Here's how the part is built. I have some questions about the finished solid (model axes, mm). A direction names the side the tool comes from. Give positions to 0.01 mm unless a question says otherwise; leave off trailing zeros. Loops run counter-clockwise (first coordinate to the right, second up) from the corner with the lowest first, then second, coordinate; pieces in that order, holes last.
Q1. I need wall thicknesses on line 1 (Y direction, x = -51, z = 2.5); line 2 (X direction, y = -1329.5, z = 13); line 3 (X direction, y = -1317.5, z = 14). Which ranges of each line are inside material? Lowest first, please.
Q2. If we section it at A-A (y = -108): Please give me the cut outline in (x, z).
Q3. We'd pull the mould along X, two halves only. Please class faces 4 (the face through (-69.85, -814, 0)), 5 (the face through (-1, -814, -19.05)), 6 (the face through (-57.15, -1588, 0)): +X half, -X half, draft (parallel to the pull), parting line (faces both ways), or undercut.
Q4. For faces 1 (the face through (31.75, -1588, 0)), 2 (the face through (-57.15, -64, 0)), 3 (the face through (69.85, -814, 0)), which set-ups out of +Z, -Z, +X, -X, +Y, -Y let a thin tool reach every point of the face, with its end or its side?
Q5. Will these pins go through, and if not, where does the flat tip stop? P1, Ø11.5, axis at x = 8, z = -4, coming from the +Y side; P2, Ø3, axis at x = 31.5, z = -8.5, coming from the +Y side; P3, Ø10, axis at x = 0.5, z = -0.5, coming from the -Y side.
Q6. If we section it at B-B (z = -1.5): Please give me the cut outline in (x, y).
Q7. If we section it at C-C (x = -33): Please give me the cut outline in (y, z).
from build123d import *

# Parameters (mm, degrees)
F1_DEPTH = 1651
F2_W     = 88.9
F2_H     = 127
F3_DEPTH = 38.101
F4_W     = 88.9
F4_H     = 127
F5_DEPTH = 38.101


with BuildPart() as f1:
    # F0 (on Front) → F1 (new body)
    with BuildSketch(Plane.XZ):
        with BuildLine():
            ThreePointArc((-69.85, -12.7), (-67.990128, -17.190128), (-63.5, -19.05))
            Line((-63.5, -19.05), (63.5, -19.05))
            ThreePointArc((63.5, -19.05), (67.990128, -17.190128), (69.85, -12.7))
            Line((69.85, -12.7), (69.85, 12.7))
            ThreePointArc((69.85, 12.7), (67.990128, 17.190128), (63.5, 19.05))
            Line((63.5, 19.05), (-63.5, 19.05))
            ThreePointArc((-63.5, 19.05), (-67.990128, 17.190128), (-69.85, 12.7))
            Line((-69.85, 12.7), (-69.85, -12.7))
        make_face()
    extrude(amount=F1_DEPTH)

    # F2 (on face) → F3 (cut, through all)
    with BuildSketch(Plane.XY.offset(19.05)):
        with Locations((-12.7, -63.5)):
            Rectangle(F2_W, F2_H)
    extrude(amount=-F3_DEPTH, mode=Mode.SUBTRACT)

    # F4 (on face) → F5 (cut, through all)
    with BuildSketch(Plane.XY.offset(19.05)):
        with Locations((-12.7, -1587.5)):
            Rectangle(F4_W, F4_H)
    extrude(amount=-F5_DEPTH, mode=Mode.SUBTRACT)


solid = f1.part
Check sheet entries:
1. line 1: y = -1524 to -127
1. line 2: x = -69.84 to 69.84
1. line 3: x = -69.72 to 69.72
2. outline: (-69.85, -12.7) arc R6.35 ccw to (-63.5, -19.05) - (-57.15, -19.05) - (-57.15, 19.05) - (-63.5, 19.05) arc R6.35 ccw to (-69.85, 12.7) - close; (31.75, -19.05) - (63.5, -19.05) arc R6.35 ccw to (69.85, -12.7) - (69.85, 12.7) arc R6.35 ccw to (63.5, 19.05) - (31.75, 19.05) - close
3. face 4: -X half
3. face 5: draft
3. face 6: undercut
4. face 1: +Z, -Z, -Y
4. face 2: +Z, -Z, +Y
4. face 3: +Z, -Z, +X, +Y, -Y
5. P1: stops at y = -127
5. P2: stops at y = 0
5. P3: stops at y = -1524
6. outline: (-69.85, -1651) - (-57.15, -1651) - (-57.15, -1524) - (31.75, -1524) - (31.75, -1651) - (69.85, -1651) - (69.85, 0) - (31.75, 0) - (31.75, -127) - (-57.15, -127) - (-57.15, 0) - (-69.85, 0) - close
7. outline: (-1524, -19.05) - (-127, -19.05) - (-127, 19.05) - (-1524, 19.05) - close
